from build123d import *

# Parameters (mm, degrees)
SKETCH1_R                = 19.05
BOSS_EXTRUDE1_DEPTH      = 15.875
BOSS_EXTRUDE2_REACH      = 290.595
BOSS_EXTRUDE2_END_RADIUS = 19.05
SKETCH3_R                = 9.525
SKETCH5_W                = 13.407996618
SKETCH5_H                = 2.54
CUT_EXTRUDE2_DEPTH       = 3.175
BOSS_EXTRUDE3_REACH      = 290.668
SKETCH6_R                = 1.27


with BuildPart() as part:
    # Sketch1 → Boss-Extrude1 (new, symmetric)
    with BuildSketch(Plane(origin=(0, 0, 0), x_dir=(1, 0, 0), z_dir=(0, 1, 0))):
        with Locations(Location((-268.478, 0, 0), (0, 0, 270))):
            Circle(SKETCH1_R)
    extrude(amount=BOSS_EXTRUDE1_DEPTH, both=True)

    # Boss-Extrude2: up to this cylinder (the profile starts outside it)
    boss_extrude2_end = Plane(origin=(-268.478, 0, 0), z_dir=(0, -1, 0)) * Cylinder(BOSS_EXTRUDE2_END_RADIUS, 620.29, mode=Mode.PRIVATE)
    # Sketch3 → Boss-Extrude2 (add, up to the surface)
    with BuildSketch(Plane(origin=(0, 0, 0), x_dir=(0, 0, -1), z_dir=(1, 0, 0)), mode=Mode.PRIVATE) as boss_extrude2_sk1:
        Circle(SKETCH3_R)
    boss_extrude2_tool1 = extrude(boss_extrude2_sk1.sketch, amount=-BOSS_EXTRUDE2_REACH, mode=Mode.PRIVATE) - boss_extrude2_end
    add(boss_extrude2_tool1.solids().sort_by_distance((0, 0, 0))[0])

    # Mirror3: part across plane


with BuildPart() as part_1:
    add(part.part)
    add(part.part.mirror(Plane(origin=(0, 0, 0), x_dir=(0, 0, 1), z_dir=(1, 0, 0))))

    # Sketch4 → Cut-Revolve1 (revolve, cut)
    with BuildSketch(Plane.XZ.offset(15.875)):
        with BuildLine():
            Line((-281.178, 0), (-255.778, 0))
            ThreePointArc((-255.778, 0), (-268.478, 12.7), (-281.178, 0))
        make_face()
        with BuildLine():
            Line((255.778, 0), (281.178, 0))
            ThreePointArc((281.178, 0), (268.478, 12.7), (255.778, 0))
        make_face()
    revolve(axis=Axis((-37.36850349, -15.875, 0), (1, 0, 0)), mode=Mode.SUBTRACT)

    # Sketch5 → Cut-Extrude2 (cut, symmetric)
    with BuildSketch(Plane(origin=(0, 0, 0), x_dir=(0, 0, -1), z_dir=(1, 0, 0))):
        with Locations((6.703998309, 0)):
            Rectangle(SKETCH5_W, SKETCH5_H)
    extrude(amount=CUT_EXTRUDE2_DEPTH, both=True, mode=Mode.SUBTRACT)

    # Sketch6 → Boss-Extrude3 (add, up to next)
    with BuildSketch(Plane(origin=(0, -1.27, 0), x_dir=(1, 0, 0), z_dir=(0, 1, 0)), mode=Mode.PRIVATE) as boss_extrude3_sk1:
        with Locations(Location((0, 6.291669235, 0), (0, 0, 90))):
            Circle(SKETCH6_R)
    boss_extrude3_tool1 = extrude(boss_extrude3_sk1.sketch, amount=BOSS_EXTRUDE3_REACH, mode=Mode.PRIVATE) - part_1.part
    add(boss_extrude3_tool1.solids().sort_by_distance((0, -1.27, -6.291669))[0])


solid = part_1.part
Read the model definition and answer for the solid it produces. Units are mm, in the model's axes. A direction names the side the tool comes from. Give positions to 0.01 mm unless a question says otherwise; leave off trailing zeros. Write each loop counter-clockwise with the first axis right and the second up, starting at its lowest first coordinate (ties: lowest second). Pieces come first, ordered by that corner, then holes. Notation, with made-up numbers: M -24.5,16.25 L -1.5,16.25 A21 cw -1.5,38.25 Z; hole C 78,-6 d6. An arc over 180 degrees is marked long. One line per item, written item: value. Start each with the question number.
(1) Find the intervals of material crossed by line 1 (X direction, y = 14, z = -9); line 2 (Y direction, x = 139.5, z = 0) (3 decimals); line 3 (X direction, y = -2, z = 11), in increasing order.
(2) Determine the mould class of faces 1 (the cylindrical face through (-287.075, 0.222, -4.13)), 2 (the flat face through (-281, -15.875, 4)) for opening direction X: pulls with the +X half, pulls with the -X half, needs draft (parallel to the pull), parting line crosses it, or undercut.
(3) A tool of negligible diameter and unlimited length cuts with its end or side. For faces 3 (the cylindrical face through (-3.528, -5.796, 7.559)), 4 (the flat face through (272.4, -15.875, 12.4)), from which of +Z, -Z, +X, -X, +Y, -Y can it reach the whole face along a straight path? Write none if from no direction.
(4) Find section A-A (x = -54). Determine the outline of the cut face in (y, z) (3 decimals), plus the area to 3 significant figures.
(5) Flat-ended cylindrical pins translate along their axes: pin 1 Ø2 at (y, z) = (0, -3.5) entering from +X; pin 2 Ø12 at (x, z) = (-160.5, 3) entering from +Y (3 decimals); pin 3 Ø10 at (y, z) = (12, 13.5) entering from -X. Find the tip coordinate at first contact, or state that the pin passes through.
Results below:
1. line 1: x = -285.27 to -251.69, 251.69 to 285.27
1. line 2: y = -9.525 to 9.525
1. line 3: x = -284.03 to -252.92, 252.92 to 284.03
2. face 1: undercut
2. face 2: needs draft
3. face 3: none
3. face 4: +Z, -Z, +X, -X, -Y
4. outline: C 0,0 d19.05
4. area: 285 mm^2
5. pin 1: stops at x = 287.36
5. pin 2: stops at y = 9.525
5. pin 3: stops at x = -285.53
